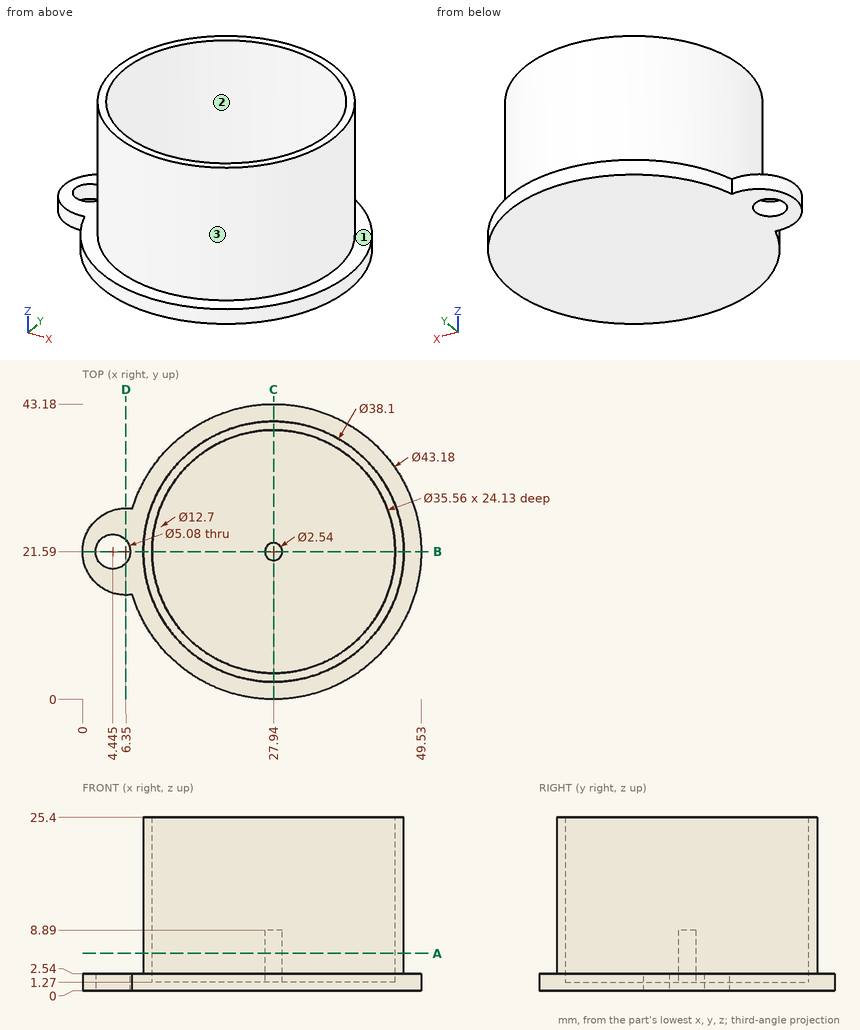
For this review, use the dimensioned drawing (mm, ordinates from the lowest corner) and the shaded views. Round coordinates to 2 decimals unless told otherwise and drop trailing zeros. Write each loop counter-clockwise with the first axis right and the second up, starting at its lowest first coordinate (ties: lowest second). Pieces come first, ordered by that corner, then holes. Notation, with made-up numbers: M -16,-34.75 L 30,-34.75 A25 cw 30,-19.75 Z; hole C 9.25,79.25 d6. An arc over 180 degrees is marked long. Answer as CSV lines item,"result". Start each with the question number.
Q1. The part is to be moulded in two halves that separate along X. For the marked faces 1, 2 and 3, say which applies: +X half, -X half, draft (parallel to the pull), parting line (faces both ways), or undercut.
Q2. Clearance check with flat-ended pins moving along their axes: P1, Ø5, axis at x = 24, z = 17, coming from the +Y side; P2, Ø3, axis at y = 20, z = 21.5, coming from the -X side; P3, Ø6, axis at x = 19, z = 12.5, coming from the -Y side. State where each tip first meets the part, or that it passes through.
Q3. Consider section A-A, the plane z = 5.5. Give the boundary of the cut face in (x, y).
Q4. Consider section B-B, the plane y = 21.59. Give the boundary of the cut face in (x, z) (3 decimals).
Q5. Consider section D-D, the plane x = 6.35. Give the boundary of the cut face in (y, z), then the cut area to 3 significant figures.
Q6. Wall thickness on line 1 along Y through (x, z) = (28.5, 10.75); line 2 along X through (y, z) = (22, 18.5); line 3 along Z through (x, y) = (25, 13.5): over which ranges is each line inside the solid? List them lowest first.
Q7. Consider section C-C, the plane x = 27.94. Give the boundary of the cut face in (y, z), then the cut area to 3 significant figures.
Result set:
1,face 1,"draft"
1,face 2,"undercut"
1,face 3,"parting line"
2,P1,"stops at y = 40.59"
2,P2,"stops at x = 8.89"
2,P3,"stops at y = 3.49"
3,outline,"C 27.94,21.59 d38.1; C 27.94,21.59 d2.54; hole C 27.94,21.59 d35.56"
4,outline,"M 0,0 L 1.905,0 L 1.905,2.54 L 0,2.54 Z; M 6.985,0 L 49.53,0 L 49.53,2.54 L 46.99,2.54 L 46.99,25.4 L 45.72,25.4 L 45.72,1.27 L 29.21,1.27 L 29.21,8.89 L 26.67,8.89 L 26.67,1.27 L 10.16,1.27 L 10.16,25.4 L 8.89,25.4 L 8.89,2.54 L 6.985,2.54 Z"
5,outline,"M 15.24,0 L 19.91,0 L 19.91,2.54 L 15.24,2.54 Z; M 23.27,0 L 27.94,0 L 27.94,2.54 L 23.27,2.54 Z"
5,area,"23.7 mm²"
6,line 1,"y = 2.55 to 3.82, 39.36 to 40.63"
6,line 2,"x = 8.89 to 10.16, 45.72 to 46.99"
6,line 3,"z = 0 to 1.27"
7,outline,"M 0,0 L 43.18,0 L 43.18,2.54 L 40.64,2.54 L 40.64,25.4 L 39.37,25.4 L 39.37,1.27 L 22.86,1.27 L 22.86,8.89 L 20.32,8.89 L 20.32,1.27 L 3.81,1.27 L 3.81,25.4 L 2.54,25.4 L 2.54,2.54 L 0,2.54 Z"
7,area,"142 mm²"
